from build123d import *

# Parameters (mm, degrees)
SKETCH2_R          = 2
SKETCH2_R_2        = 1.5
CUT_EXTRUDE1_DEPTH = 12
CHAMFER1_SIZE      = 0.3
SKETCH3_R          = 1.5
CUT_EXTRUDE2_DEPTH = 6


with BuildPart() as part:
    # Sketch1 → Revolve1 (revolve)
    with BuildSketch(Plane.XY, mode=Mode.PRIVATE) as revolve1_sk:
        Polygon((-6, 0), (6, 0), (6, 11), (4, 11), (4, 5), (-6, 5), align=None)
    revolve(revolve1_sk.sketch.rotate(Axis((-6, 0, 0), (1, 0, 0)), 90), axis=Axis((-6, 0, 0), (1, 0, 0)))

    # Sketch2 → Cut-Extrude1 (cut)
    with BuildSketch(Plane.ZY.offset(6)):
        Circle(SKETCH2_R)
        with Locations((-5.656854249, 5.656854249)):
            Circle(SKETCH2_R_2)
        with Locations((5.656854249, 5.656854249)):
            Circle(SKETCH2_R_2)
        with Locations((5.656854249, -5.656854249)):
            Circle(SKETCH2_R_2)
        with Locations((-5.656854249, -5.656854249)):
            Circle(SKETCH2_R_2)
    extrude(amount=-CUT_EXTRUDE1_DEPTH, mode=Mode.SUBTRACT)

    # Chamfer1
    chamfer1_edges = [part.edges().sort_by_distance(p)[0] for p in [
        (6, -5.656854249, -7.156854249),
        (4, -5.656854249, -7.156854249),
        (6, -5.656854249, 4.156854249),
        (4, -5.656854249, 4.156854249),
        (6, 5.656854249, 4.156854249),
        (4, 5.656854249, 4.156854249),
        (6, 5.656854249, -7.156854249),
        (4, 5.656854249, -7.156854249),
        (6, 0, -2),
        (-6, 0, -2),
        (4, 0, -5),
        (4, 0, -11),
        (6, 0, -11),
        (-6, 0, -5),
    ]]
    chamfer(chamfer1_edges, length=CHAMFER1_SIZE)

    # Sketch3 → Cut-Extrude2 (cut, symmetric)
    with BuildSketch(Plane.XY):
        with Locations((-2, 0)):
            Circle(SKETCH3_R)
    extrude(amount=CUT_EXTRUDE2_DEPTH, both=True, mode=Mode.SUBTRACT)


solid = part.part
Could you check a few things on this model? Use its own coordinates, in mm. A direction names the side the tool comes from. Round coordinates to 2 decimals unless told otherwise and drop trailing zeros. Loops run counter-clockwise (first coordinate to the right, second up) from the corner with the lowest first, then second, coordinate; pieces in that order, holes last. Notation, with made-up numbers: (-1, 14) -> (23, 14) arc R26 cw to (23, 44) -> close; hole circle Ø4 at (17, 15). An arc over 180 degrees is marked (long way). Use CSV: the item, a comma, the result in double quotes.
(1) If I drill on probe 1 along Y at (x, z) = (5.25, -4.5); probe 2 along X at (y, z) = (-3, -4.5); probe 3 along X at (y, z) = (0, 3.5), over which ranges is the centre line in solid material (lowest first)? Write a range as [from, to].
Return value:
probe 1,"y = [-10.04, -6.61], [-4.7, 4.7], [6.61, 10.04]"
probe 2,"x = [4, 6]"
probe 3,"x = [-6, -3.5], [-0.5, 6]"
(2) Suppose I cut it at B-B on z = 0. Write out the boundary of the cut face in (x, y).
Return value:
outline,"(-6, -4.7) -> (-5.7, -5) -> (3.7, -5) -> (4, -5.3) -> (4, -10.7) -> (4.3, -11) -> (5.7, -11) -> (6, -10.7) -> (6, -2.3) -> (5.7, -2) -> (-5.7, -2) -> (-6, -2.3) -> close; (-6, 2.3) -> (-5.7, 2) -> (5.7, 2) -> (6, 2.3) -> (6, 10.7) -> (5.7, 11) -> (4.3, 11) -> (4, 10.7) -> (4, 5.3) -> (3.7, 5) -> (-5.7, 5) -> (-6, 4.7) -> close"
(3) Suppose I cut it at D-D on x = 1.75. Write out the boundary of the cut face in (y, z), plus the area to 3 significant figures.
Return value:
outline,"circle Ø10 at (0, 0); hole circle Ø4 at (0, 0)"
area,"66.0 mm²"
(4) For faces 1 (the cylindrical face through (-0.08, 1.686, 1.075)), 2 (the flat face through (4, -5, -3)), which set-ups out of +Z, -Z, +X, -X, +Y, -Y let a thin tool reach every point of the face, with its end or its side?
Return value:
face 1,"+X, -X"
face 2,"-X"
(5) Will these pins go through, and if not, where does the flat tip stop? pin 1 Ø1 at (x, y) = (1, 3.5) entering from +Z; pin 2 Ø1 at (x, y) = (3, 3) entering from +Z; pin 3 Ø5 at (y, z) = (5.66, -5.66) entering from -X.
Return value:
pin 1,"stops at z = 4"
pin 2,"stops at z = 4.33"
pin 3,"stops at x = 4"
(6) Suppose I cut it at C-C on x = -2. Write out the boundary of the cut face in (y, z), plus the area to 3 significant figures.
Return value:
outline,"(-1.5, -4.77) -> (-1.5, -1.32) arc R2 cw to (-1.5, 1.32) -> (-1.5, 4.77) arc R5 ccw to start; (1.5, -4.77) arc R5 ccw to (1.5, 4.77) -> (1.5, 1.32) arc R2 cw to (1.5, -1.32) -> close"
area,"47.2 mm²"
(7) If we mould it in two halves opening along Y, with no side actions, what happens to faces 3 (the cylindrical face through (4.99, 10.74, -2.38)), 4 (the cylindrical face through (4.99, 4.193, -5.982)), 5 (the flat face through (6, -3, 0))? For each: +Y half, -Y half, draft (parallel to the pull), parting line (faces both ways), or undercut.
Return value:
face 3,"parting line"
face 4,"undercut"
face 5,"draft"
(8) Suppose I cut it at A-A on y = 0. Give the number of separate pieces and of enclosed holes in the cut face, plus the area to 3 significant figures.
Return value:
separate pieces,"4"
enclosed holes,"0"
area,"77.6 mm²"
